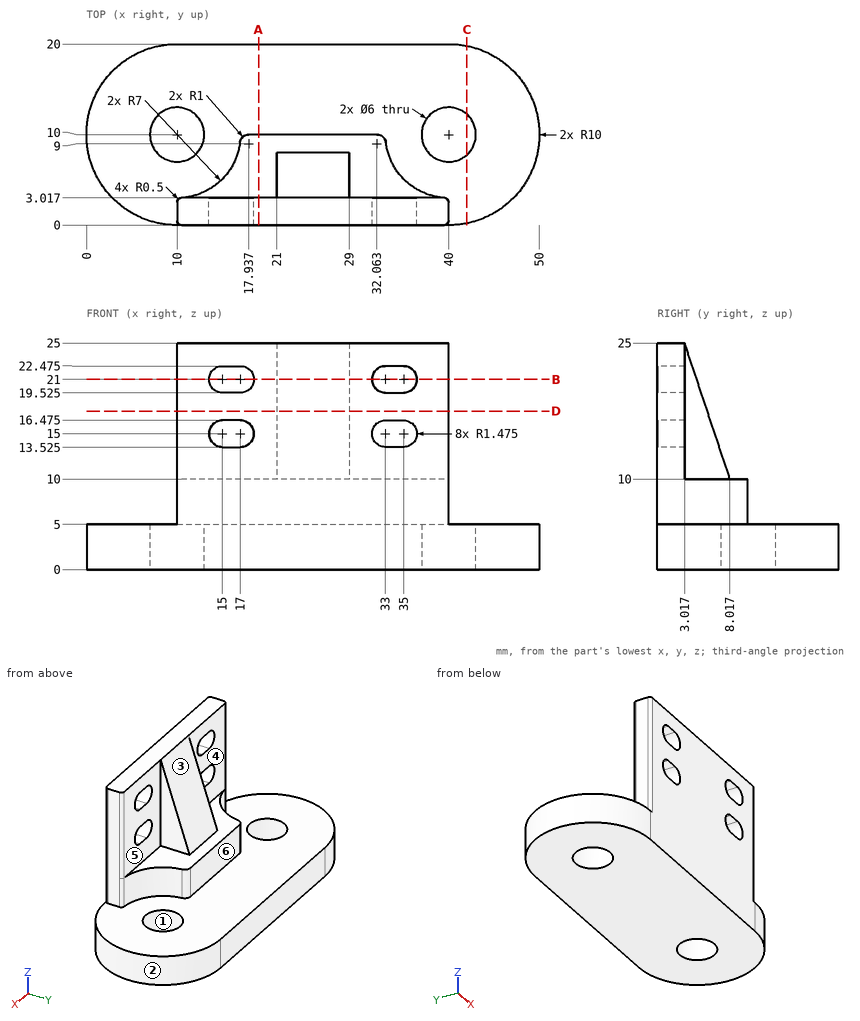
Input: dimensioned drawing with shaded views. Units: mm. Origin: part minimum x, y, z. A direction names the side the tool comes from. Give positions to 0.01 mm unless a question says otherwise; leave off trailing zeros. Write each loop counter-clockwise with the first axis right and the second up, starting at its lowest first coordinate (ties: lowest second). Pieces come first, ordered by that corner, then holes. Notation, with made-up numbers: M 73,11 L 86,11 A18 cw 86,17 Z; hole C 32.5,17.5 d6. An arc over 180 degrees is marked long. Return JSON: item names as keys, results as strings. Group by question number.
1) Cut plane A-A, the plane x = 19. Output: boundary loops of the cut face in (y, z), plus the area to 3 significant figures.
2) Pull-direction query (X, two-part tool) for the marked faces 1, 2 and 3; classes: pulls with the +X half, pulls with the -X half, needs draft (parallel to the pull), parting line crosses it, or undercut.
3) Cut plane D-D, the plane z = 17.5. Output: boundary loops of the cut face in (x, y), plus the area to 3 significant figures.
4) Set-up query: the marked faces 4, 5 and 6. Return all of +Z, -Z, +X, -X, +Y, -Y with unobstructed straight access to the full face (end or side cutting, diameter ignored); none if empty.
5) Pin query (flat end, axial travel): P1, Ø1.6, axis at x = 16.5, y = 1, coming from the -Z side; P2, Ø4, axis at y = 5.5, z = 16, coming from the +X side; P3, Ø0.6, axis at y = 1.5, z = 14.5, coming from the -X side; P4, Ø8.5, axis at x = 34.5, z = 18.5, coming from the +Y side. Return the tip coordinate at first contact, or that it passes through.
6) Material intervals for line 1 along Y through (x, z) = (10, 2.1); line 2 along X through (y, z) = (8.5, 4); line 3 along Y through (x, z) = (16, 13.25), sorted ascending. Write a range as [from, to].
7) Cut plane C-C, the plane x = 42. Output: boundary loops of the cut face in (y, z).
8) Cut plane B-B, the plane z = 21. Give the number of separate pieces and of enclosed holes in the cut face.
Recorded:
{
 "1": {"outline": "M 0,0 L 20,0 L 20,5 L 10,5 L 10,10 L 3.02,10 L 3.02,25 L 0,25 Z", "area": "195 mm²"},
 "2": {"face 1": "undercut", "face 2": "pulls with the +X half", "face 3": "needs draft"},
 "3": {"outline": "M 10,0.5 A0.5 ccw 10.5,0 L 39.5,0 A0.5 ccw 40,0.5 L 40,2.52 A0.5 ccw 39.5,3.02 L 29,3.02 L 29,5.52 L 21,5.52 L 21,3.02 L 10.5,3.02 A0.5 ccw 10,2.52 Z", "area": "110 mm²"},
 "4": {"face 4": "+Z, -X, +Y", "face 5": "+Z, +X, +Y", "face 6": "+Z, +X, -X, +Y"},
 "5": {"P1": "stops at z = 0", "P2": "stops at x = 29", "P3": "stops at x = 10", "P4": "stops at y = 3.02"},
 "6": {"line 1": "y = [0, 7], [13, 20]", "line 2": "x = [0.11, 7.4], [12.6, 37.4], [42.6, 49.89]", "line 3": "y = [0, 3.02]"},
 "7": {"outline": "M 0.2,0 L 7.76,0 L 7.76,5 L 0.2,5 Z; M 12.24,0 L 19.8,0 L 19.8,5 L 12.24,5 Z"},
 "8": {"separate pieces": "3", "enclosed holes": "0"}
}
